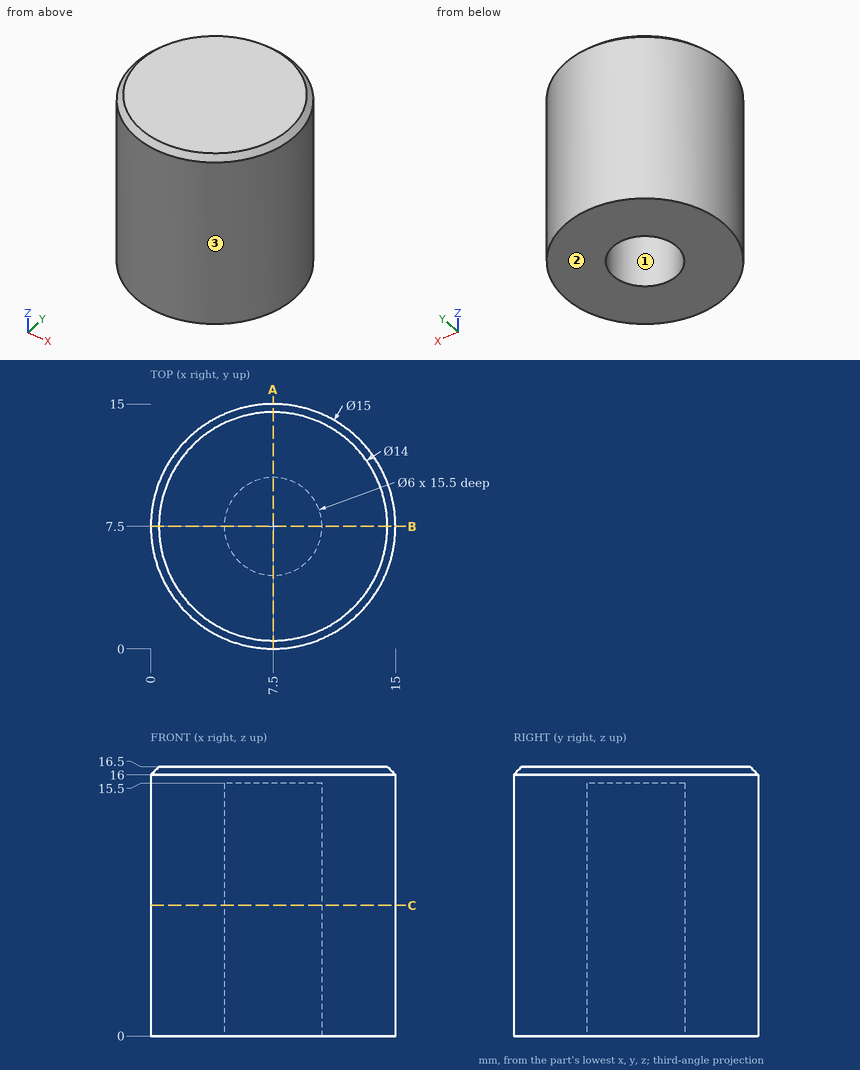
Part print with two shaded views. Sizes in mm from the minimum x, y, z corner. Coordinates: 2 decimals unless noted, no trailing zeros. Write each loop counter-clockwise with the first axis right and the second up, starting at its lowest first coordinate (ties: lowest second). Pieces come first, ordered by that corner, then holes. Notation, with made-up numbers: M 58.25,64.25 L 95.25,64.25 A27 cw 95.25,84.25 Z; hole C 26,74 d8. An arc over 180 degrees is marked long. Return JSON: item names as keys, results as strings.
Item 1: Slice it at A-A, the plane x = 7.5. Write the cut outline in (y, z), and give its area (3 significant figures).
Findings below:
{"outline": "M 0,0 L 4.5,0 L 4.5,15.5 L 10.5,15.5 L 10.5,0 L 15,0 L 15,16 L 14.5,16.5 L 0.5,16.5 L 0,16 Z", "area": "154 mm2"}
Item 2: Two-plate mould, pull along Y, no slides. Class the marked faces 1, 2 and 3: +Y half, -Y half, draft (parallel to the pull), parting line (faces both ways), or undercut.
Findings below:
{"face 1": "undercut", "face 2": "draft", "face 3": "parting line"}
Item 3: Probe line 1 (Y direction, x = 7.5, z = 4); line 2 (Z direction, x = 7, y = 10); line 3 (X direction, y = 7, z = 9.75). List the from-to ranges inside material, lowest first. Write a range as from..to.
Findings below:
{"line 1": "y = 0..4.5, 10.5..15", "line 2": "z = 15.5..16.5", "line 3": "x = 0.02..4.54, 10.46..14.98"}
Item 4: Slice it at C-C, the plane z = 8. Write the cut outline in (x, y), and give its area (3 significant figures).
Findings below:
{"outline": "C 7.5,7.5 d15; hole C 7.5,7.5 d6", "area": "148 mm2"}
Item 5: Drop flat-ended pins along their axis: pin 1 Ø1 at (x, z) = (12, 3.5) entering from -Y; pin 2 Ø8 at (x, z) = (12.5, 13) entering from +Y; pin 3 Ø2 at (x, z) = (5, 7) entering from +Y. Give the stop position or say it passes through.
Findings below:
{"pin 1": "stops at y = 1.16", "pin 2": "stops at y = 14.93", "pin 3": "stops at y = 14.85"}
